```python
from build123d import *

# Parameters (mm, degrees)
F0_R          = 63.5
F0_R_2        = 38.1
F1_DEPTH      = 31.75
F4_DEPTH      = 8.89
F9_D          = 8.89
F11_DEPTH     = 8.89
F13_D         = 8.89
F14_T4_DEPTH  = 114.3
F14_S6_R      = 25.2026770054
F14_T7_DEPTH  = 59
F14_T11_DEPTH = 114.3
F14_S13_R     = 25.2026770054
F14_T14_DEPTH = 59
F14_T18_DEPTH = 114.3
F14_S20_R     = 25.2026770054
F14_T21_DEPTH = 59
F14_T25_DEPTH = 114.3
F14_S27_R     = 25.2026770054
F14_T28_DEPTH = 59
F14_T32_DEPTH = 114.3
F14_S34_R     = 25.2026770054
F14_T35_DEPTH = 59
F14_T39_DEPTH = 114.3
F14_S41_R     = 25.2026770054
F14_T42_DEPTH = 59
F14_T46_DEPTH = 114.3
F14_S48_R     = 25.2026770054
F14_T49_DEPTH = 59
F14_S54_R     = 2.54
F14_T55_DEPTH = 99
F14_S56_R     = 2.54
F14_T57_DEPTH = 99


# Not quite as in the source:
# - a fillet or chamfer that OpenCascade refuses, or shapes differently, is made with other operations: its cross-section is extruded or revolved along the edge and cut away or added
# - a feature of the source that left no trace in its solid (it failed there, or was rolled back) is left out


with BuildPart() as f1:
    # F0 (on Top) → F1 (new body)
    with BuildSketch(Plane.XY):
        Circle(F0_R)
        Circle(F0_R_2, mode=Mode.SUBTRACT)
    extrude(amount=F1_DEPTH)

    # F3 (on offset) → F4 (join)
    with BuildSketch(Plane.XZ.offset(38.1)):
        with BuildLine():
            Line((-25.2026770054, 119.2994092428), (-40.64, 31.75))
            Line((-40.64, 31.75), (40.64, 31.75))
            Line((40.64, 31.75), (25.2026770054, 119.2994092428))
            ThreePointArc((25.2026770054, 119.2994092428), (0, 144.5020862482), (-25.2026770054, 119.2994092428))
        make_face()
    extrude(amount=F4_DEPTH)

    # F9 (through all)
    with Locations(Plane.XZ.offset(46.99)):
        with Locations((0, 119.2994092428)):
            Hole(F9_D / 2)

    # F6 (on offset) → F11 (join)
    with BuildSketch(Plane.XZ.offset(-38.1)):
        with BuildLine():
            Line((-25.2026770054, 119.2994092428), (-40.64, 31.75))
            Line((-40.64, 31.75), (40.64, 31.75))
            Line((40.64, 31.75), (25.2026770054, 119.2994092428))
            ThreePointArc((25.2026770054, 119.2994092428), (0, 144.5020862482), (-25.2026770054, 119.2994092428))
        make_face()
    extrude(amount=-F11_DEPTH)

    # F13 (through all)
    with Locations(Plane(origin=(0, 46.99, 0), x_dir=(-1, 0, 0), z_dir=(0, 1, 0))):
        with Locations((0, 119.2994092428)):
            Hole(F13_D / 2)

    # F14: fillet of radius 2.54 on 8 edges, made by hand


with BuildPart() as f14_tool2:
    # F14_s3 → F14_t4 (new body)
    with BuildSketch(Plane(origin=(22.9494446088, 0, 130.1527679803), x_dir=(0, 1, 0), z_dir=(-0.1736481777, 0, -0.984807753))):
        with BuildLine():
            ThreePointArc((-46.99, -42.9959167233), (-46.2460512242, -44.7919679476), (-44.45, -45.5359167233))
            Line((-44.45, -45.5359167233), (-46.99, -45.5359167233))
            Line((-46.99, -45.5359167233), (-46.99, -42.9959167233))
        make_face()
    extrude(amount=F14_T4_DEPTH)

    split(bisect_by=Plane.XY.offset(31.75), keep=Keep.TOP)

    # F14_s6 → F14_t7 (cut, symmetric)
    with BuildSketch(Plane.XZ.offset(45.7)):
        with Locations((0, 119.2994092428)):
            Circle(F14_S6_R)
    extrude(amount=F14_T7_DEPTH, both=True, mode=Mode.SUBTRACT)


with BuildPart() as f1_1:
    add(f1.part)

    # F14_t1: cut F14_tool2
    add(f14_tool2.part, mode=Mode.SUBTRACT)


with BuildPart() as f14_tool9:
    # F14_s10 → F14_t11 (new body)
    with BuildSketch(Plane(origin=(-3.1014579015, 0, 17.589241811), x_dir=(0, 1, 0), z_dir=(-0.1736481777, 0, 0.984807753))):
        with BuildLine():
            ThreePointArc((-46.99, -42.9959167233), (-46.2460512242, -44.7919679476), (-44.45, -45.5359167233))
            Line((-44.45, -45.5359167233), (-46.99, -45.5359167233))
            Line((-46.99, -45.5359167233), (-46.99, -42.9959167233))
        make_face()
    extrude(amount=F14_T11_DEPTH)

    split(bisect_by=Plane.XY.offset(31.75), keep=Keep.TOP)

    # F14_s13 → F14_t14 (cut, symmetric)
    with BuildSketch(Plane.XZ.offset(45.7)):
        with Locations((0, 119.2994092428)):
            Circle(F14_S13_R)
    extrude(amount=F14_T14_DEPTH, both=True, mode=Mode.SUBTRACT)


with BuildPart() as f1_2:
    add(f1_1.part)

    # F14_t8: cut F14_tool9
    add(f14_tool9.part, mode=Mode.SUBTRACT)


with BuildPart() as f14_tool16:
    # F14_s17 → F14_t18 (new body)
    with BuildSketch(Plane(origin=(22.9494446088, 0, 130.1527679803), x_dir=(0, 1, 0), z_dir=(-0.1736481777, 0, -0.984807753))):
        with BuildLine():
            ThreePointArc((-40.64, -45.5359167233), (-38.8439487758, -44.7919679476), (-38.1, -42.9959167233))
            Line((-38.1, -42.9959167233), (-38.1, -45.5359167233))
            Line((-38.1, -45.5359167233), (-40.64, -45.5359167233))
        make_face()
    extrude(amount=F14_T18_DEPTH)

    split(bisect_by=Plane.XY.offset(31.75), keep=Keep.TOP)

    # F14_s20 → F14_t21 (cut, symmetric)
    with BuildSketch(Plane.XZ.offset(39.4)):
        with Locations((0, 119.2994092428)):
            Circle(F14_S20_R)
    extrude(amount=F14_T21_DEPTH, both=True, mode=Mode.SUBTRACT)


with BuildPart() as f1_3:
    add(f1_2.part)

    # F14_t15: cut F14_tool16
    add(f14_tool16.part, mode=Mode.SUBTRACT)


with BuildPart() as f14_tool23:
    # F14_s24 → F14_t25 (new body)
    with BuildSketch(Plane(origin=(-3.1014579015, 0, 17.589241811), x_dir=(0, 1, 0), z_dir=(-0.1736481777, 0, 0.984807753))):
        with BuildLine():
            ThreePointArc((40.64, -45.5359167233), (38.8439487758, -44.7919679476), (38.1, -42.9959167233))
            Line((38.1, -42.9959167233), (38.1, -45.5359167233))
            Line((38.1, -45.5359167233), (40.64, -45.5359167233))
        make_face()
    extrude(amount=F14_T25_DEPTH)

    split(bisect_by=Plane.XY.offset(31.75), keep=Keep.TOP)

    # F14_s27 → F14_t28 (cut, symmetric)
    with BuildSketch(Plane.XZ.offset(-39.4)):
        with Locations((0, 119.2994092428)):
            Circle(F14_S27_R)
    extrude(amount=F14_T28_DEPTH, both=True, mode=Mode.SUBTRACT)


with BuildPart() as f1_4:
    add(f1_3.part)

    # F14_t22: cut F14_tool23
    add(f14_tool23.part, mode=Mode.SUBTRACT)


with BuildPart() as f14_tool30:
    # F14_s31 → F14_t32 (new body)
    with BuildSketch(Plane(origin=(-3.1014579015, 0, 17.589241811), x_dir=(0, 1, 0), z_dir=(-0.1736481777, 0, 0.984807753))):
        with BuildLine():
            ThreePointArc((44.45, -45.5359167233), (46.2460512242, -44.7919679476), (46.99, -42.9959167233))
            Line((46.99, -42.9959167233), (46.99, -45.5359167233))
            Line((46.99, -45.5359167233), (44.45, -45.5359167233))
        make_face()
    extrude(amount=F14_T32_DEPTH)

    split(bisect_by=Plane.XY.offset(31.75), keep=Keep.TOP)

    # F14_s34 → F14_t35 (cut, symmetric)
    with BuildSketch(Plane.XZ.offset(-45.7)):
        with Locations((0, 119.2994092428)):
            Circle(F14_S34_R)
    extrude(amount=F14_T35_DEPTH, both=True, mode=Mode.SUBTRACT)


with BuildPart() as f1_5:
    add(f1_4.part)

    # F14_t29: cut F14_tool30
    add(f14_tool30.part, mode=Mode.SUBTRACT)


with BuildPart() as f14_tool37:
    # F14_s38 → F14_t39 (new body)
    with BuildSketch(Plane(origin=(22.9494446088, 0, 130.1527679803), x_dir=(0, 1, 0), z_dir=(-0.1736481777, 0, -0.984807753))):
        with BuildLine():
            ThreePointArc((46.99, -42.9959167233), (46.2460512242, -44.7919679476), (44.45, -45.5359167233))
            Line((44.45, -45.5359167233), (46.99, -45.5359167233))
            Line((46.99, -45.5359167233), (46.99, -42.9959167233))
        make_face()
    extrude(amount=F14_T39_DEPTH)

    split(bisect_by=Plane.XY.offset(31.75), keep=Keep.TOP)

    # F14_s41 → F14_t42 (cut, symmetric)
    with BuildSketch(Plane.XZ.offset(-45.7)):
        with Locations((0, 119.2994092428)):
            Circle(F14_S41_R)
    extrude(amount=F14_T42_DEPTH, both=True, mode=Mode.SUBTRACT)


with BuildPart() as f1_6:
    add(f1_5.part)

    # F14_t36: cut F14_tool37
    add(f14_tool37.part, mode=Mode.SUBTRACT)


with BuildPart() as f14_tool44:
    # F14_s45 → F14_t46 (new body)
    with BuildSketch(Plane(origin=(22.9494446088, 0, 130.1527679803), x_dir=(0, 1, 0), z_dir=(-0.1736481777, 0, -0.984807753))):
        with BuildLine():
            ThreePointArc((40.64, -45.5359167233), (38.8439487758, -44.7919679476), (38.1, -42.9959167233))
            Line((38.1, -42.9959167233), (38.1, -45.5359167233))
            Line((38.1, -45.5359167233), (40.64, -45.5359167233))
        make_face()
    extrude(amount=F14_T46_DEPTH)

    split(bisect_by=Plane.XY.offset(31.75), keep=Keep.TOP)

    # F14_s48 → F14_t49 (cut, symmetric)
    with BuildSketch(Plane.XZ.offset(-39.4)):
        with Locations((0, 119.2994092428)):
            Circle(F14_S48_R)
    extrude(amount=F14_T49_DEPTH, both=True, mode=Mode.SUBTRACT)


with BuildPart() as f1_7:
    add(f1_6.part)

    # F14_t43: cut F14_tool44
    add(f14_tool44.part, mode=Mode.SUBTRACT)


with BuildPart() as f14_tool51:
    # F14_s52 → F14_t53 (revolve)
    with BuildSketch(Plane.XZ):
        with BuildLine():
            ThreePointArc((63.5, 29.21), (62.7560512242, 31.0060512242), (60.96, 31.75))
            Line((60.96, 31.75), (63.5, 31.75))
            Line((63.5, 31.75), (63.5, 29.21))
        make_face()
    revolve(axis=Axis((0, 0, 31.75), (0, 0, 1)))

    # F14_s54 → F14_t55 (cut, symmetric)
    with BuildSketch(Plane(origin=(5.20944533, 0, 29.5442325904), x_dir=(0, 1, 0), z_dir=(0.1736481777, 0, 0.984807753))):
        with Locations((-44.45, 42.9959167233)):
            Circle(F14_S54_R)
    extrude(amount=F14_T55_DEPTH, both=True, mode=Mode.SUBTRACT)

    # F14_s56 → F14_t57 (cut, symmetric)
    with BuildSketch(Plane(origin=(-5.20944533, 0, 29.5442325904), x_dir=(0, 1, 0), z_dir=(0.1736481777, 0, -0.984807753))):
        with Locations((-44.45, 42.9959167233)):
            Circle(F14_S56_R)
    extrude(amount=F14_T57_DEPTH, both=True, mode=Mode.SUBTRACT)


with BuildPart() as f1_8:
    add(f1_7.part)

    # F14_t50: cut F14_tool51
    add(f14_tool51.part, mode=Mode.SUBTRACT)


solid = f1_8.part
```
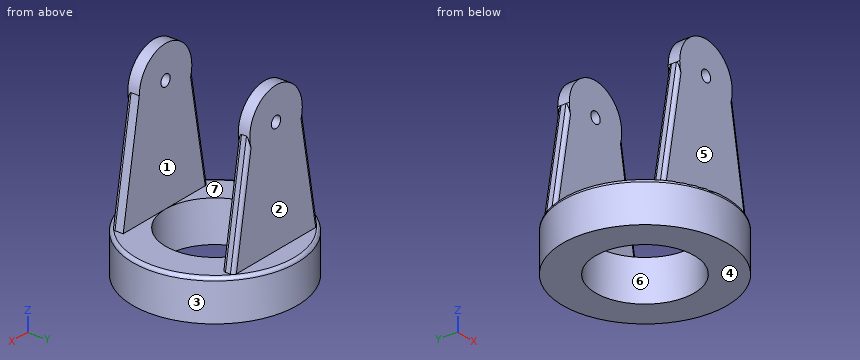
Build history of the part. All positions in model axes, mm. Face numbers are marked on the shaded views. A direction names the side the tool comes from. Round coordinates to 2 decimals unless told otherwise and drop trailing zeros. Loops run counter-clockwise (first coordinate to the right, second up) from the corner with the lowest first, then second, coordinate; pieces in that order, holes last.
Item 1: Which spindle directions (+Z, -Z, +X, -X, +Y, -Y) get a long thin tool onto all of the face, cutting with end or side? Do the marked faces 1, 2 and 3. Say none if no direction does.
Item 2: Two-plate mould, pull along Y, no slides. Class the marked faces 4, 5, 6 and 7: released by +Y, released by -Y, zero draft, split by the parting line, or undercut.
Item 3: Pin check, flat tips, straight feed: P1, Ø6, axis at x = 16.5, y = 49, coming from the +Z side; P2, Ø10, axis at x = 42.5, z = 28, coming from the -Y side; P3, Ø1, axis at x = 8, y = 50, coming from the +Z side. Stop position of each tip, or through.
Item 4: Saw through at A-A (y = 0). List the corners of the cut face in (x, z).
Item 5: Drill centre lines: line 1 along Y through (x, z) = (-5.5, 55.5); line 2 along Z through (x, y) = (0, 41); line 3 along Z through (x, y) = (-6.5, 49). Where is each one in solid material? Low to high.
Worked answers:
1. face 1: +Z, +X, -X
1. face 2: +Z, +X, -X, +Y
1. face 3: +Z, -Z
2. face 4: zero draft
2. face 5: released by -Y
2. face 6: undercut
2. face 7: undercut
3. P1: stops at z = 140.07
3. P2: stops at y = -51.24
3. P3: stops at z = 31.75
4. outline: (-63.5, 0) - (-38.1, 0) - (-38.1, 31.75) - (-60.96, 31.75) arc R2.54 ccw to (-63.5, 29.21) - close; (38.1, 0) - (63.5, 0) - (63.5, 29.21) arc R2.54 ccw to (60.96, 31.75) - (38.1, 31.75) - close
5. line 1: y = -46.99 to -38.1, 38.1 to 46.99
5. line 2: z = 0 to 114.85, 123.74 to 144.5
5. line 3: z = 0 to 31.75
